Geometry check sheet. Reference: the model listing, model coordinates, mm. Face numbers are marked on the shaded views. A direction names the side the tool comes from. Coordinates: 2 decimals unless noted, no trailing zeros. Loops run counter-clockwise (first coordinate to the right, second up) from the corner with the lowest first, then second, coordinate; pieces in that order, holes last.
Autodesk Inventor part; units mm, degrees
ref_plane "YZ Plane" through (0, 0, 0) normal (1, 0, 0) x (0, 1, 0)
ref_plane "XZ Plane" through (0, 0, 0) normal (0, 1, 0) x (-1, 0, 0)
ref_plane "XY Plane" through (0, 0, 0) normal (0, 0, 1) x (1, 0, 0)
sketch "Sketch1" plane through (0, 0, 0) normal (0, 1, 0) x (-1, 0, 0)
  line L0 (5, 12.5) -> (-5, 12.5)
  line L1 (-5, 12.5) -> (-5, -12.5)
  line L2 (-5, -12.5) -> (5, -12.5)
  line L3 (5, -12.5) -> (5, 12.5)
  line L4 (5, 12.5) -> (-5, -12.5) construction
  line L5 (-5, 12.5) -> (5, -12.5) construction
  line L6 (0, 7.5) -> (0, -7.5) construction
  line L7 (-1.5875, 7.5) -> (-1.5875, -7.5)
  line L8 (1.5875, -7.5) -> (1.5875, 7.5)
  arc A0 (1.5875, 7.5) -> (-1.5875, 7.5) centre (0, 7.5) ccw
  arc A1 (-1.5875, -7.5) -> (1.5875, -7.5) centre (0, -7.5) ccw
  point P0 (0, 0)
  point P1 (0, 0)
  dimension "d0" = 10
  dimension "d1" = 25
  dimension "d2" = 7.5
  dimension "d3" = 7.5
  dimension "d4" = 3.175
extrude "Extrusion1" add sketch "Sketch1" along normal blind 2
sketch "Sketch2" plane through (0, 2, 0) normal (0, 1, 0) x (1, 0, 0)
  line L0 (5, -12.5) -> (5, 12.5)
  line L1 (5, 12.5) -> (-5, 12.5)
  line L2 (-5, 12.5) -> (-5, -12.5)
  line L3 (-5, -12.5) -> (5, -12.5)
  arc A0 (-1.5875, -7.5) -> (1.5875, -7.5) centre (0, -7.5) ccw
  line L4 (-1.5875, -7.5) -> (-1.5875, 7.5)
  arc A1 (1.5875, 7.5) -> (-1.5875, 7.5) centre (0, 7.5) ccw
  line L5 (1.5875, 7.5) -> (1.5875, -7.5)
  line L6 (-3, -10.5) -> (-3, 10.5)
  line L7 (3, 10.5) -> (3, -10.5)
  line L8 (3, -10.5) -> (-3, -10.5)
  line L9 (-3, 10.5) -> (-3, 12.5)
  line L10 (3, 10.5) -> (3, 12.5)
  point P0 (0, 0)
  dimension "d7" = 2
sketch "Sketch3" plane through (0, 0, 0) normal (1, 0, 0) x (0, 1, 0)
  line L0 (2, 12.5) -> (26.198, 36.698)
  point P0 (0, 0)
  dimension "d15" = 34.2211
sweep "Sweep1" add profiles "Sketch2" path "Sketch3" contours L3 L2 L1 L9 L6 L8 L7 L10 L0
chamfer "Chamfer1" distance 2 angle 45 1 edges at (0, 0, 12.5)
sketch "Sketch5" plane through (-5, 26.198, 36.698) normal (0, 1, 0) x (1, 0, 0)
  line L0 (20, 0) -> (-10, 0)
  line L1 (-10, 0) -> (-10, 25)
  line L2 (-10, 25) -> (20, 25)
  line L3 (20, 25) -> (20, 0)
  line L4 (10, 0) -> (10, 25)
  circle A0 centre (15, 12.5) radius 2.5
  circle A1 centre (-5, 12.5) radius 2.5
  point P0 (5, 36.698)
  dimension "d23" = 25
  dimension "d24" = 30
  dimension "d25" = 10
  dimension "d26" = 5
  dimension "d27" = 5
  dimension "d28" = 5
  dimension "d29" = 5
extrude "Extrusion4" add sketch "Sketch5" along normal blind 2
fillet "Fillet1" radius 10 4 edges at (15, 27.198, 11.698) (-15, 27.198, 11.698) (-15, 27.198, 36.698) (15, 27.198, 36.698)
properties part number "ancla"
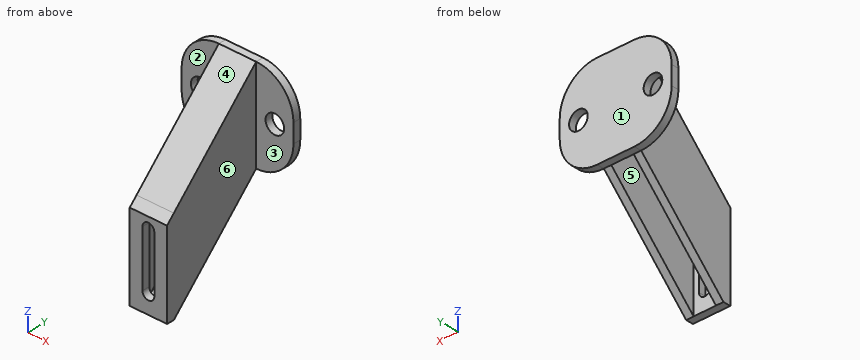
1) Section check C-C on z = 29. Record the cut outline in (x, y), and give its area (3 significant figures).
Data:
outline: (-14.73, 26.2) - (-5, 26.2) - (-5, 18.5) - (5, 18.5) - (5, 26.2) - (14.73, 26.2) - (14.73, 28.2) - (-14.73, 28.2) - close; hole (-3, 20.5) - (3, 20.5) - (3, 26.2) - (-3, 26.2) - close
area: 102 mm2
2) Section check D-D on y = 4.5. Record the cut outline in (x, z).
Data:
outline: (-5, -10) - (-3, -10) - (-3, 13) - (3, 13) - (3, -10) - (5, -10) - (5, 15) - (-5, 15) - close
3) Material ranges on probe 1 along X at (y, z) = (25.25, 13); probe 2 along Y at (x, z) = (-1.5, 10); probe 3 along Z at (x, y) = (-10, 27.1), recorded low to high.
Data:
probe 1: x = -5 to -3, 3 to 5
probe 2: y = 0 to 2
probe 3: z = 13.04 to 21.7, 26.7 to 35.36
4) Section check B-B on x = -10. Record the cut outline in (y, z).
Data:
outline: (26.2, 13.04) - (28.2, 13.04) - (28.2, 21.7) - (26.2, 21.7) - close; (26.2, 26.7) - (28.2, 26.7) - (28.2, 35.36) - (26.2, 35.36) - close
5) Section check A-A on z = -5. Record the cut outline in (x, y), and give its area (4 significant figures).
Data:
outline: (-5, 0) - (-1.59, 0) - (-1.59, 2) - (-3, 2) - (-3, 9.5) - (-5, 9.5) - close; (1.59, 0) - (5, 0) - (5, 9.5) - (3, 9.5) - (3, 2) - (1.59, 2) - close
area: 43.65 mm2
6) Access from +Z, -Z, +X, -X, +Y, -Y to the whole of each face (thin tool, end or side, straight path). Record for the marked faces 1, 2 and 3.
Data:
face 1: +Z, -Z, +X, -X, +Y
face 2: +Z, -Z, -X, -Y
face 3: +Z, -Z, +X, -Y
7) Mould release check, pull along X, two halves, no side actions. Record for the marked faces 4, 5 and 6: +X half, -X half, draft (parallel to the pull), parting line (faces both ways), or undercut.
Data:
face 4: draft
face 5: undercut
face 6: +X half
8) Depth check by flat-ended pin: pin 1 (12 mm diameter, centred on y = 11, z = 9, fed in from -X); pin 2 (6 mm diameter, centred on x = -1, z = -4.5, fed in from +Y); pin 3 (2 mm diameter, centred on x = 3, z = -6.5, fed in from +Y); pin 4 (4.5 mm diameter, centred on x = 10, z = 24.198, fed in from +Y). Enter the tip coordinate at first touch or a pass-through.
Data:
pin 1: stops at x = -5
pin 2: stops at y = 12.24
pin 3: stops at y = 9
pin 4: passes through
